CAD build for the part. Positions are in the model's coordinates, mm. A direction names the side the tool comes from. Give positions to 0.01 mm unless a question says otherwise; leave off trailing zeros. Loops run counter-clockwise (first coordinate to the right, second up) from the corner with the lowest first, then second, coordinate; pieces in that order, holes last. Notation, with made-up numbers: M 21.25,77 L 32.25,77 A8 ccw 32.25,92 Z; hole C 17,72.25 d1. An arc over 180 degrees is marked long. Answer as CSV lines item,"result".
Autodesk Inventor part; units mm, degrees
ref_plane "YZ Plane" through (0, 0, 0) normal (1, 0, 0) x (0, 1, 0)
ref_plane "XZ Plane" through (0, 0, 0) normal (0, 1, 0) x (-1, 0, 0)
ref_plane "XY Plane" through (0, 0, 0) normal (0, 0, 1) x (1, 0, 0)
sketch "Sketch1" plane through (0, 0, 0) normal (0, 0, 1) x (1, 0, 0)
  line L0 (-7.7614, 0) -> (138.2386, 0)
  line L1 (138.2386, 0) -> (138.2386, 29.6)
  line L2 (-7.7614, 29.6) -> (-7.7614, 0)
  line L3 (-7.7614, 29.6) -> (22.1386, 29.6)
  line L4 (12.489, 18.1) -> (114.8883, 18.1)
  line L5 (22.1386, 29.6) -> (12.489, 18.1)
  line L6 (22.1386, 29.6) -> (41.4586, 29.6) construction
  line L7 (138.2386, 29.6) -> (105.2386, 29.6)
  line L8 (105.2386, 29.6) -> (114.8883, 18.1)
  point P0 (0, 0)
  dimension "d0" = 146
  dimension "d1" = 29.6
  dimension "d2" = 29.9
  dimension "d4" = 130
  dimension "d5" = 33
  dimension "d6" = 50
extrude "Extrusion1" add sketch "Sketch1" against normal blind 486
sketch "Sketch2" plane through (-7.7614, 29.6, 0) normal (0, 1, 0) x (1, 0, 0)
  line L0 (113, 0) -> (122.6496, 0)
  line L1 (124, 486) -> (113, 0)
  line L2 (113, 0) -> (113, 486)
  line L3 (113, 486) -> (124, 486)
  line L4 (122.6496, 0) -> (122.6496, 486)
  line L5 (113, 486) -> (113, 0)
  line L6 (146, 0) -> (146, 486)
  point P0 (7.7614, 0)
  dimension "d9" = 22
sketch "Sketch3" plane through (-7.7614, 0, 0) normal (0, -1, 0) x (1, 0, 0)
  line L0 (20.2504, -486) -> (122.6496, -486)
  line L1 (0, 0) -> (146, 0)
  circle A0 centre (71.6943, -409.4001) radius 62.1
  line L2 (71.45, -486) -> (71.4962, -471.5001)
  circle A1 centre (71.6943, -409.4001) radius 52
  circle A2 centre (71.6943, -409.4001) radius 9.51
  circle A3 centre (72.1613, -247.2004) radius 4.1
  point P0 (7.7614, 0)
  dimension "d10" = 124.2
  dimension "d11" = 14.5
  dimension "d12" = 62.1
  dimension "d13" = 104
  dimension "d14" = 19.02
  dimension "d15" = 8.2
extrude "Extrusion2" cut sketch "Sketch3" against normal blind 13 contours A0
extrude "Extrusion3" add sketch "Sketch3" along normal blind 7.5 contours A2
extrude "Extrusion4" cut sketch "Sketch3" against normal through all contours A3
sketch "Sketch4" plane through (12.489, 18.1, 0) normal (0, 1, 0) x (1, 0, 0)
  circle A0 centre (51.911, 247.2004) radius 4.1
  circle A1 centre (51.911, 247.2004) radius 9.5
  line L0 (0, 486) -> (102.3993, 486)
  line L1 (51.1996, 486) -> (51.1996, 476.6)
  arc A2 (46.6496, 476.6) -> (46.6496, 457.9) centre (46.6496, 467.25) ccw
  arc A3 (55.7496, 457.9) -> (55.7496, 476.6) centre (55.7496, 467.25) ccw
  line L2 (46.6496, 476.6) -> (55.7496, 476.6)
  line L3 (46.6496, 457.9) -> (55.7496, 457.9)
  circle A4 centre (51.1996, 411.4) radius 8.5
  point P0 (-12.489, 0)
  point P1 (51.1996, 476.6)
  dimension "d23" = 19
  dimension "d26" = 9.4
  dimension "d29" = 0
  dimension "d30" = 18.7
  dimension "d31" = 18.7
  dimension "d38" = 17
  dimension "d39" = 46.5
extrude "Extrusion5" cut sketch "Sketch4" against normal blind 3.7 contours A1
extrude "Extrusion7" cut sketch "Sketch4" against normal blind 6 contours L2 A3 L3 A2
extrude "Extrusion8" cut sketch "Sketch4" against normal blind 3 contours A4
sketch "Sketch5" plane through (-7.7614, 0, 0) normal (0, -1, 0) x (1, 0, 0)
  point P0 (7.7614, 0)
sketch "Sketch6" plane through (-7.7614, 0, 0) normal (0, -1, 0) x (1, 0, 0)
  circle A0 centre (86, -261) radius 5
  line L0 (146, -486) -> (0, -486)
  line L1 (146, 0) -> (146, -486)
  circle A1 centre (60.5, -235.5) radius 5.5
  line L2 (0, 0) -> (0, -486)
  circle A2 centre (134.5, -295.5) radius 5.5
  point P0 (7.7614, 0)
  dimension "d42" = 10
  dimension "d43" = 225
  dimension "d44" = 60
  dimension "d45" = 11
  dimension "d46" = 60.5
  dimension "d47" = 250.5
  dimension "d48" = 11
  dimension "d49" = 190.5
  dimension "d50" = 11.5
hole "Hole1" at (126.7386, 0, -295.5) direction (0, 1, 0) diameter 8.5 end through all counterbore diameter 11 counterbore depth 8.5
hole "Hole2" at (78.2386, 0, -261) direction (0, 1, 0) diameter 7 end through all counterbore diameter 10 counterbore depth 7.5
hole "Hole3" at (52.7386, 0, -235.5) direction (0, 1, 0) diameter 7.5 end through all counterbore diameter 11 counterbore depth 7
thread "Thread1"
properties part number "slide ontop of saddle"
1) Band-saw the part on D-D on x = 99. Give the cut face in (y, z).
Answer below:
outline,"M 0,-486 L 18.1,-486 L 18.1,0 L 0,0 L 0,-358.15 L 13,-358.15 L 13,-371 L 0,-371 L 0,-447.8 L 13,-447.8 L 13,-460.65 L 0,-460.65 Z"
2) Mould opens along X. For faces 1 (the face through (7, 29.6, -240)), 2 (the face through (-7.761, 15, -240)), 3 (the face through (131, 8.5, -297)) say: +X half, -X half, draft (parallel to the pull), parting line (faces both ways), or undercut.
Answer below:
face 1,"draft"
face 2,"-X half"
face 3,"undercut"
3) Band-saw the part on B-B on z = -148.5. Give the cut face in (x, y), and give its area (3 significant figures).
Answer below:
outline,"M -7.76,0 L 138.24,0 L 138.24,29.6 L 105.24,29.6 L 114.89,18.1 L 12.49,18.1 L 22.14,29.6 L -7.76,29.6 Z"
area,"3,250 mm^2"
4) Which spindle directions (+Z, -Z, +X, -X, +Y, -Y) get a long thin tool onto all of the face, cutting with end or side? Do faces 4 (the face through (52, 18.1, -240)), 5 (the face through (125.087, 4.31, -300.746)), 6 (the face through (126.552, 19.198, -291.254)), 7 (the face through (62.341, 16.276, -237.926)). Say none if no direction does.
Answer below:
face 4,"+Z, -Z"
face 5,"-Y"
face 6,"+Y, -Y"
face 7,"+Y"
5) Band-saw the part on C-C on x = 33. Give the cut face in (y, z).
Answer below:
outline,"M 0,-486 L 18.1,-486 L 18.1,0 L 0,0 L 0,-355.55 L 13,-355.55 L 13,-367.6 L 0,-367.6 L 0,-451.2 L 13,-451.2 L 13,-463.25 L 0,-463.25 Z"
6) Band-saw the part on A-A on z = -295.5. Give the cut face in (x, y).
Answer below:
outline,"M -7.76,0 L 121.24,0 L 121.24,8.5 L 122.49,8.5 L 122.49,29.6 L 105.24,29.6 L 114.89,18.1 L 12.49,18.1 L 22.14,29.6 L -7.76,29.6 Z; M 130.99,8.5 L 132.24,8.5 L 132.24,0 L 138.24,0 L 138.24,29.6 L 130.99,29.6 Z"
7) Flat gauge pins, fed straight in: pin 1 (3 mm diameter, centred on x = 93, z = -391, fed in from -Y); pin 2 (21 mm diameter, centred on x = 65.5, z = -242.5, fed in from +Y); pin 3 (3 mm diameter, centred on x = 67, z = -460.5, fed in from +Y). Where does each tip first touch, or does it go through?
Answer below:
pin 1,"stops at y = 0"
pin 2,"stops at y = 18.1"
pin 3,"stops at y = 12.1"
8) Drill centre lines: line 1 (Z direction, x = 64.4, y = 17.2); line 2 (Z direction, x = 105.5, y = 2.5); line 3 (Z direction, x = 21, y = 4). Where is each one in solid material? Low to high. Write a range as from..to.
Answer below:
line 1,"z = -486..-476.6, -457.9..-419.87, -402.93..-256.7, -237.7..0"
line 2,"z = -486..-455.54, -440.64..-378.16, -363.26..0"
line 3,"z = -486..-454.27, -438.74..-380.06, -364.53..0"
